Design review of the part shown in the three views and the two pictorial views. Dimensions are in mm from the part's minimum x, y and z. A direction names the side the tool comes from. Give positions to 0.01 mm unless a question says otherwise; leave off trailing zeros. Write each loop counter-clockwise with the first axis right and the second up, starting at its lowest first coordinate (ties: lowest second). Pieces come first, ordered by that corner, then holes. Notation, with made-up numbers: M 59.5,85.25 L 87.5,85.25 A14 cw 87.5,107.25 Z; hole C -11,7 d2. An arc over 180 degrees is marked long. Write item = value, one per line.
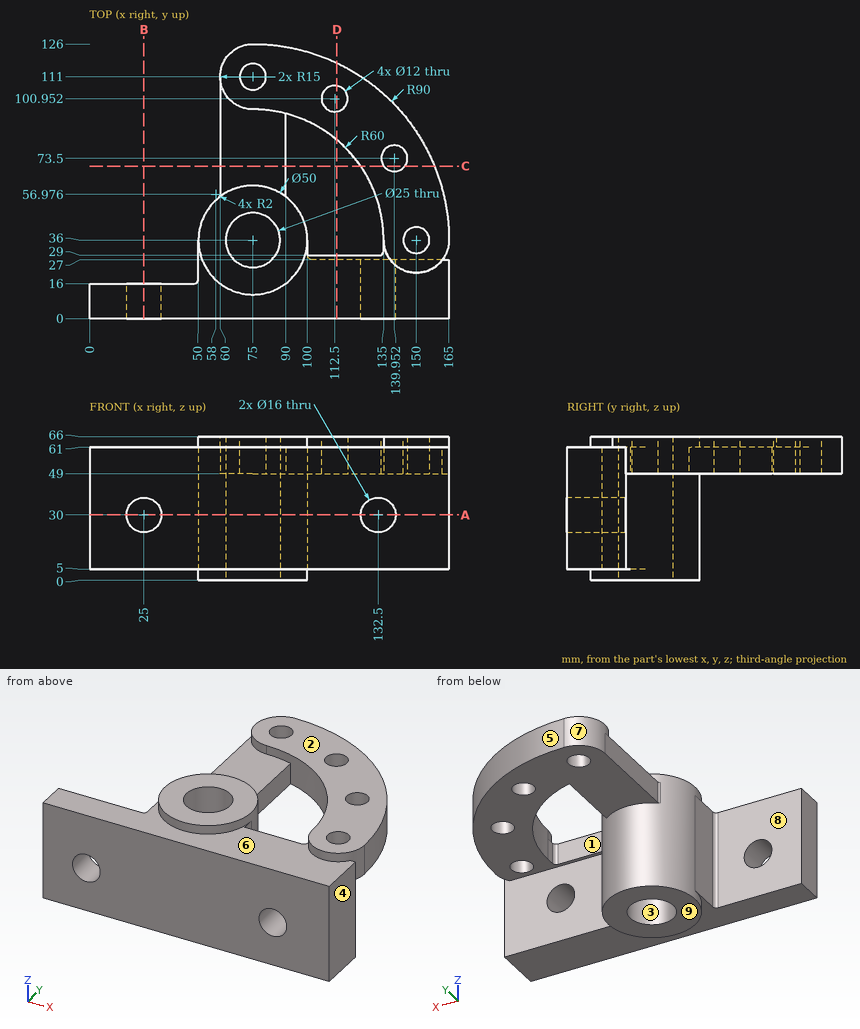
1. Machinability: for the marked faces 5, 6, 7, 8 and 9, which of the approach directions +Z, -Z, +X, -X, +Y, -Y give a long, thin tool a straight path to every point of the face, cutting with its end or side? Answer none if there is none.
Responses:
face_5 = +Z, -Z, +X, +Y
face_6 = +Z, -Y
face_7 = +Z, -X
face_8 = +Z, -Z, -X, +Y
face_9 = -Z, +X, -X, +Y, -Y
2. We need section A-A, the plane z = 30. Write out the cut boundary in (x, y).
Responses:
outline = M 0,0 L 17,0 L 17,16 L 0,16 Z; M 33,0 L 124.5,0 L 124.5,27 L 102,27 A2 cw 100,29 L 100,36 A25 ccw 50,36 L 50,18 A2 cw 48,16 L 33,16 Z; M 140.5,0 L 165,0 L 165,27 L 140.5,27 Z; hole C 75,36 d25
3. Insertion check: P1, Ø10, axis at x = 118, z = 58, coming from the +Y side; P2, Ø3.5, axis at y = 74, z = 55, coming from the +X side; P3, Ø5, axis at x = 98.5, z = 30.5, coming from the +Y side (1 decimal). Each pin has a flat end and moves straight along its axis. Give the tip position at first contact, or say it passes through.
Responses:
P1 = 117.58
P2 = 157.38
P3 = 49.6
4. The part is to be moulded in two halves that separate along X. For the marked faces 1, 2, 3 and 4, say which applies: +X half, -X half, draft (parallel to the pull), parting line (faces both ways), or undercut.
Responses:
face_1 = undercut
face_2 = draft
face_3 = undercut
face_4 = +X half
5. We need section D-D, the plane x = 113.5. Write out the cut boundary in (y, z), then the cut area to 3 significant figures.
Responses:
outline = M 0,5 L 27,5 L 27,49 L 29,49 L 29,61 L 0,61 Z; M 82.02,49 L 95.04,49 L 95.04,66 L 82.02,66 Z; M 106.87,49 L 117.35,49 L 117.35,66 L 106.87,66 Z
area = 1,940 mm2
6. For line 1 along Y through (x, z) = (75, 60.5); line 2 along Y through (x, z) = (126.5, 44); line 3 along Y through (x, z) = (8, 35.5), list the stretches that pass through material, from the lowest coordinate up. Write a range as from..to.
Responses:
line_1 = 0..23.5, 48.5..105, 117..126
line_2 = 0..27
line_3 = 0..16
7. We need section C-C, the plane y = 70. Write out the cut boundary in (x, z) (1 decimal).
Responses:
outline = M 60,49 L 90,49 L 90,61 L 60,61 Z; M 124.4,49 L 135.1,49 L 135.1,66 L 124.4,66 Z; M 144.8,49 L 158.3,49 L 158.3,66 L 144.8,66 Z
8. We need section B-B, the plane x = 25. Write out the cut boundary in (y, z).
Responses:
outline = M 0,5 L 16,5 L 16,22 L 0,22 Z; M 0,38 L 16,38 L 16,61 L 0,61 Z
